```python
from build123d import *

# Parameters (mm, degrees)
SKETCH_1_R               = 8
EXTRUDE_1_DEPTH          = 22
CUT_EXTRUDE_1_DEPTH      = 25.738633754
CUT_EXTRUDE_1_DEPTH_BACK = 25.738633754
CUT_EXTRUDE_2_DEPTH      = 26
CUT_EXTRUDE_2_DEPTH_BACK = 26
SKETCH_3_R               = 2
CUT_EXTRUDE_3_DEPTH      = 26
CUT_EXTRUDE_3_DEPTH_BACK = 26
SKETCH_4_W               = 8
SKETCH_4_H               = 8
SKETCH_5_R               = 4
CUT_EXTRUDE_4_DEPTH      = 9
CUT_EXTRUDE_5_DEPTH      = 25.738633907
CUT_EXTRUDE_5_DEPTH_BACK = 25.738633907
SKETCH_6_R               = 1.5


with BuildPart() as part:
    # Sketch 1 → Extrude 1 (new body)
    with BuildSketch(Plane.XY):
        Circle(SKETCH_1_R)
    extrude(amount=EXTRUDE_1_DEPTH)

    # Sketch 2 → Cut-Extrude 1 (cut, two sides: drawn at the far end of the back side and taken through both)
    with BuildSketch(Plane(origin=(0, 0, 0), x_dir=(1, 0, 0), z_dir=(0, 1, 0)).offset(-CUT_EXTRUDE_1_DEPTH_BACK)):
        with BuildLine():
            Line((8, -9), (4, -13))
            Line((4, -13), (4, -18))
            ThreePointArc((4, -18), (0, -22), (-4, -18))
            Line((-4, -18), (-4, -13))
            Line((-4, -13), (-8, -9))
            Line((-8, -9), (-8, -22))
            Line((-8, -22), (1.483160763, -24.700219192))
            Line((1.483160763, -24.700219192), (8, -22))
            Line((8, -22), (8, -9))
        make_face()
    extrude(amount=CUT_EXTRUDE_1_DEPTH + CUT_EXTRUDE_1_DEPTH_BACK, mode=Mode.SUBTRACT)

    # Sketch 3 → Cut-Extrude 2 (cut, two sides: drawn at the far end of the back side and taken through both)
    with BuildSketch(Plane(origin=(0, 0, 0), x_dir=(1, 0, 0), z_dir=(0, 1, 0)).offset(-CUT_EXTRUDE_2_DEPTH_BACK)):
        with Locations(Location((0, -18, 0), (0, 0, 270))):
            Circle(SKETCH_3_R)
    extrude(amount=CUT_EXTRUDE_2_DEPTH + CUT_EXTRUDE_2_DEPTH_BACK, mode=Mode.SUBTRACT)

    # Sketch 4 → Cut-Extrude 3 (cut, two sides: drawn at the far end of the back side and taken through both)
    with BuildSketch(Plane(origin=(0, 0, 0), x_dir=(0, 0, -1), z_dir=(1, 0, 0)).offset(-CUT_EXTRUDE_3_DEPTH_BACK)):
        with Locations((-18, 0)):
            Rectangle(SKETCH_4_W, SKETCH_4_H)
    extrude(amount=CUT_EXTRUDE_3_DEPTH + CUT_EXTRUDE_3_DEPTH_BACK, mode=Mode.SUBTRACT)

    # Sketch 5 → Cut-Extrude 4 (cut)
    with BuildSketch(Plane(origin=(0, 0, 0), x_dir=(-1, 0, 0), z_dir=(0, 0, -1))):
        Circle(SKETCH_5_R)
    extrude(amount=-CUT_EXTRUDE_4_DEPTH, mode=Mode.SUBTRACT)

    # Sketch 6 → Cut-Extrude 5 (cut, two sides: drawn at the far end of the back side and taken through both)
    with BuildSketch(Plane(origin=(0, 0, 0), x_dir=(0, 0, -1), z_dir=(1, 0, 0)).offset(-CUT_EXTRUDE_5_DEPTH_BACK)):
        with Locations((-5, 0)):
            Circle(SKETCH_6_R)
    extrude(amount=CUT_EXTRUDE_5_DEPTH + CUT_EXTRUDE_5_DEPTH_BACK, mode=Mode.SUBTRACT)


solid = part.part
```
The model under review builds one solid part; all positions refer to its coordinate system, in mm. A direction names the side the tool comes from. Coordinates: 2 decimals unless noted, no trailing zeros. Write each loop counter-clockwise with the first axis right and the second up, starting at its lowest first coordinate (ties: lowest second). Pieces come first, ordered by that corner, then holes. Notation, with made-up numbers: (-11, 8.25) -> (41, 8.25) arc R17 cw to (41, 26.25) -> close; hole circle Ø4 at (28.5, -37.75). An arc over 180 degrees is marked (long way). One line per item, written item: value. Start each with the question number.
Q1. Add section B-B, the plane y = 0. Give the boundary of the cut face in (x, z), then the cut area to 3 significant figures.
Q2. Add section C-C, the plane z = 17.25. Give the boundary of the cut face in (x, y).
Q3. To check wall thickness, follow probe 1 along X at (y, z) = (6.15, 18); probe 2 along Y at (x, z) = (1.75, 15); probe 3 along Z at (x, y) = (6.75, 0). State the ranges of each line that lie inside material, in increasing order.
Q4. Clearance check with flat-ended pins moving along their axes: P1, Ø1, axis at x = 1, z = 4.5, coming from the -Y side; P2, Ø5.5, axis at y = -2.5, z = 16, coming from the +X side; P3, Ø3, axis at x = -2, z = 17.5, coming from the -Y side. State where each tip first meets the part, or that it passes through.
Q5. The part is to be moulded in two halves that separate along Z. For faces 1 (the face through (0, -6, 22)), 2 (the face through (5.82, 0.07, 6.5)), 3 (the face through (2, -6, 18)), 4 (the face through (4, -0.1, 13.8)), say which applies: +Z half, -Z half, draft (parallel to the pull), parting line (faces both ways), or undercut.
Q6. For faces 5 (the face through (6, 0, 11)), 6 (the face through (-4, -0.1, 13.3)), 7 (the face through (-1.846, -3.549, 4.437)), 8 (the face through (-2, 4, 17)), 9 (the face through (0, 6, 22)), list the 3-axis set-ups (+Z, -Z, +X, -X, +Y, -Y) from which the entire face can be reached by the end or side of a thin tool; tool diameter is ignored.
Q7. Add section D-D, the plane z = 5. Give the boundary of the cut face in (x, y).
Q8. Add section A-A, the plane x = 0. Give the boundary of the cut face in (y, z), then the cut area to 3 significant figures.
Response:
1. outline: (-8, 0) -> (-4, 0) -> (-4, 3.5) -> (-8, 3.5) -> close; (-8, 6.5) -> (-4, 6.5) -> (-4, 9) -> (4, 9) -> (4, 6.5) -> (8, 6.5) -> (8, 9) -> (4, 13) -> (4, 14) -> (-4, 14) -> (-4, 13) -> (-8, 9) -> close; (4, 0) -> (8, 0) -> (8, 3.5) -> (4, 3.5) -> close
1. area: 104 mm²
2. outline: (-4, -6.93) arc R8 ccw to (-1.85, -7.78) -> (-1.85, -4) -> (-4, -4) -> close; (-4, 4) -> (-1.85, 4) -> (-1.85, 7.78) arc R8 ccw to (-4, 6.93) -> close; (1.85, -7.78) arc R8 ccw to (4, -6.93) -> (4, -4) -> (1.85, -4) -> close; (1.85, 4) -> (4, 4) -> (4, 6.93) arc R8 ccw to (1.85, 7.78) -> close
3. probe 1: -4 to -2, 2 to 4
3. probe 2: -7.81 to -4, 4 to 7.81
3. probe 3: 0 to 3.5, 6.5 to 10.25
4. P1: y = -7.98
4. P2: x = 4
4. P3: y = -7.93
5. face 1: +Z half
5. face 2: undercut
5. face 3: undercut
5. face 4: draft
6. face 5: +Z, +X, +Y, -Y
6. face 6: +Z, -X, +Y, -Y
6. face 7: -Z
6. face 8: +Z, +X, -X
6. face 9: +Z, +Y, -Y
7. outline: (-7.86, -1.5) arc R8 ccw to (7.86, -1.5) -> (3.71, -1.5) arc R4 cw to (-3.71, -1.5) -> close; (-7.86, 1.5) -> (-3.71, 1.5) arc R4 cw to (3.71, 1.5) -> (7.86, 1.5) arc R8 ccw to start
8. outline: (-8, 0) -> (-4, 0) -> (-4, 9) -> (4, 9) -> (4, 0) -> (8, 0) -> (8, 16) -> (4, 16) -> (4, 14) -> (-4, 14) -> (-4, 16) -> (-8, 16) -> close; (-8, 20) -> (-4, 20) -> (-4, 22) -> (-8, 22) -> close; (4, 20) -> (8, 20) -> (8, 22) -> (4, 22) -> close
8. area: 184 mm²
